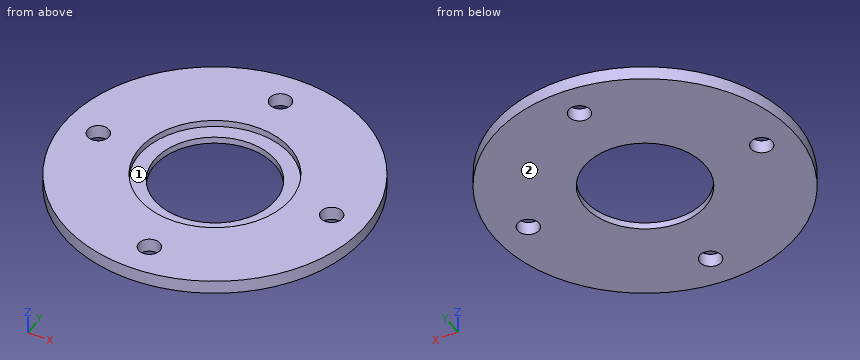
from build123d import *

# Parameters (mm, degrees)
SKETCH_1_R               = 22.5
SKETCH_1_R_2             = 9
EXTRUDE_1_DEPTH          = 2
SKETCH_2_R               = 1.6
CUT_EXTRUDE_1_DEPTH      = 3
PATTERN_CIRCULAR_2_COUNT = 4
SKETCH_3_R               = 11.25
SKETCH_3_R_2             = 9
CUT_EXTRUDE_2_DEPTH      = 1


with BuildPart() as part:
    # ｽｹｯﾁ1 → ﾎﾞｽ - 押し出し1 (new body)
    with BuildSketch(Plane.XY):
        Circle(SKETCH_1_R)
        Circle(SKETCH_1_R_2, mode=Mode.SUBTRACT)
    extrude(amount=EXTRUDE_1_DEPTH)

    # ｽｹｯﾁ2 → ｶｯﾄ - 押し出し1 (cut, through all)
    with BuildSketch(Plane.XY.offset(2)):
        with Locations((-17.5, 0)):
            Circle(SKETCH_2_R)
    cut_extrude_1 = extrude(amount=-CUT_EXTRUDE_1_DEPTH, mode=Mode.SUBTRACT)

    # 円形ﾊﾟﾀｰﾝ2: ｶｯﾄ - 押し出し1 ×4 about axis
    pattern_circular_2_axis = Axis((0, 0, 0), (0, 0, 1))
    for i in range(1, PATTERN_CIRCULAR_2_COUNT):
        add(cut_extrude_1.rotate(pattern_circular_2_axis, i * 360 / PATTERN_CIRCULAR_2_COUNT), mode=Mode.SUBTRACT)

    # ｽｹｯﾁ3 → ｶｯﾄ - 押し出し2 (cut)
    with BuildSketch(Plane.XY.offset(2)):
        Circle(SKETCH_3_R)
        Circle(SKETCH_3_R_2, mode=Mode.SUBTRACT)
    extrude(amount=-CUT_EXTRUDE_2_DEPTH, mode=Mode.SUBTRACT)


solid = part.part
Input: part model. Units: mm. Frame: model coordinates. Face numbers are marked on the shaded views. Give positions to 0.01 mm unless a question says otherwise; leave off trailing zeros. Write each loop counter-clockwise with the first axis right and the second up, starting at its lowest first coordinate (ties: lowest second). Pieces come first, ordered by that corner, then holes.
Q1. Material intervals for probe 1 along X at (y, z) = (8, 1.1); probe 2 along Y at (x, z) = (-10, 1.25); probe 3 along Y at (x, z) = (5.5, 0.35), sorted ascending.
Q2. Pull-direction query (Z, two-part tool) for the marked faces 1 and 2; classes: pulls with the +Z half, pulls with the -Z half, needs draft (parallel to the pull), parting line crosses it, or undercut.
Q3. First-contact query: P1, Ø1.9, axis at x = 0, y = -17.5, coming from the +Z side. Flat tip, straight axial feed; report the tip coordinate or a pass-through.
Q4. Section D-D, the plane x = -8. Output: boundary loops of the cut face in (y, z), plus the area to 3 significant figures.
Q5. Section A-A, the plane x = 0. Output: boundary loops of the cut face in (y, z), plus the area to 3 significant figures.
Q6. Section C-C, the plane z = 0.55. Output: boundary loops of the cut face in (x, y), plus the area to 3 significant figures.
Filled in:
1. probe 1: x = -21.03 to -7.91, 7.91 to 21.03
1. probe 2: y = -20.16 to -5.15, 5.15 to 20.16
1. probe 3: y = -21.82 to -7.12, 7.12 to 21.82
2. face 1: pulls with the +Z half
2. face 2: pulls with the -Z half
3. P1: passes through
4. outline: (-21.03, 0) - (-4.12, 0) - (-4.12, 1) - (-7.91, 1) - (-7.91, 2) - (-21.03, 2) - close; (4.12, 0) - (21.03, 0) - (21.03, 2) - (7.91, 2) - (7.91, 1) - (4.12, 1) - close
4. area: 60.1 mm2
5. outline: (-22.5, 0) - (-19.1, 0) - (-19.1, 2) - (-22.5, 2) - close; (-15.9, 0) - (-9, 0) - (-9, 1) - (-11.25, 1) - (-11.25, 2) - (-15.9, 2) - close; (9, 0) - (15.9, 0) - (15.9, 2) - (11.25, 2) - (11.25, 1) - (9, 1) - close; (19.1, 0) - (22.5, 0) - (22.5, 2) - (19.1, 2) - close
5. area: 36.7 mm2
6. outline: circle Ø45 at (0, 0); hole circle Ø3.2 at (-17.5, 0); hole circle Ø18 at (0, 0); hole circle Ø3.2 at (0, -17.5); hole circle Ø3.2 at (0, 17.5); hole circle Ø3.2 at (17.5, 0)
6. area: 1,300 mm2
